The drawing under review shows one solid part. Ordinate dimensions are in mm from its lowest x, y, z. A direction names the side the tool comes from. Round coordinates to 2 decimals unless told otherwise and drop trailing zeros. Order: outer loops, then holes, each group sorted by start corner. A loop starts at its lowest first (then second) coordinate and runs counter-clockwise, first axis right, second up.
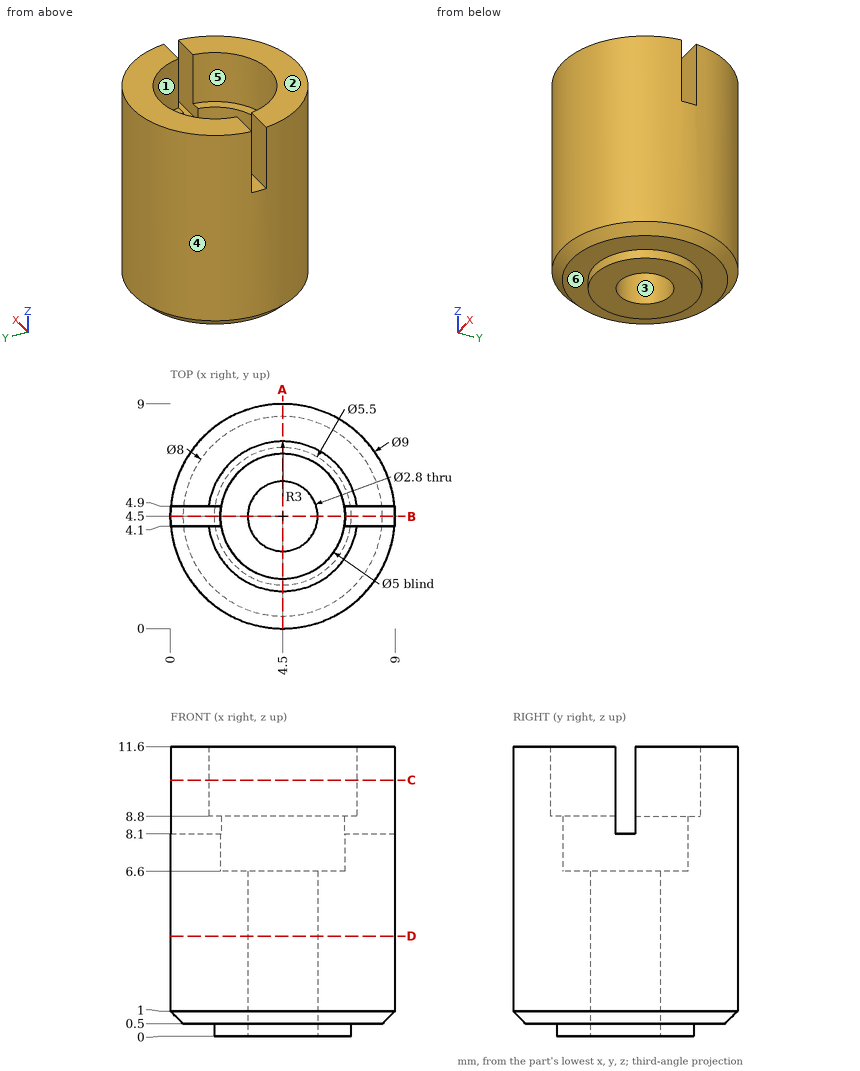
Q1. Wall thickness on line 1 (Y direction, x = 4.5, z = 7.5); line 2 (Y direction, x = 4.5, z = 3): over which ranges is each line inside the solid? List them lowest first.
Q2. Mouldability with a two-part tool opening along X and no side actions: class the marked faces 3, 4, 5 and 6 as +X half, -X half, draft (parallel to the pull), parting line (faces both ways), or undercut.
Q3. Take a section at B-B, the plane y = 4.5. State the section outline as (x, z) points.
Q4. Take a section at A-A, the plane x = 4.5. State the section outline as (y, z) points, plus the area to 3 significant figures.
Q5. Clearance check with flat-ended pins moving along their axes: pin 1 (1 mm diameter, centred on x = 8, z = 9, fed in from -Y); pin 2 (4 mm diameter, centred on y = 2.5, z = 9.5, fed in from +X); pin 3 (1.3 mm diameter, centred on x = 4.5, y = 3.5, fed in from +Z); pin 4 (1.5 mm diameter, centred on x = 4.5, y = 4, fed in from +Z). State where each tip first meets the part, or that it passes through.
Q6. Tool access review of the marked faces 1 and 2: name each direction out of +Z, -Z, +X, -X, +Y, -Y from which nothing blocks a thin tool from reaching the whole face with its end or side.
Q7. Take a section at D-D, the plane z = 4. State the section outline as (x, y) points.
Q8. Take a section at C-C, the plane z = 10.25. State the section outline as (x, y) points.
Working result:
1. line 1: y = 0 to 2, 7 to 9
1. line 2: y = 0 to 3.1, 5.9 to 9
2. face 3: undercut
2. face 4: parting line
2. face 5: undercut
2. face 6: draft
3. outline: (0, 1) - (0.5, 0.5) - (1.75, 0.5) - (1.75, 0) - (3.1, 0) - (3.1, 6.6) - (2, 6.6) - (2, 8.1) - (0, 8.1) - close; (5.9, 0) - (7.25, 0) - (7.25, 0.5) - (8.5, 0.5) - (9, 1) - (9, 8.1) - (7, 8.1) - (7, 6.6) - (5.9, 6.6) - close
4. outline: (0, 1) - (0.5, 0.5) - (1.75, 0.5) - (1.75, 0) - (3.1, 0) - (3.1, 6.6) - (2, 6.6) - (2, 8.8) - (1.5, 8.8) - (1.5, 11.6) - (0, 11.6) - close; (5.9, 0) - (7.25, 0) - (7.25, 0.5) - (8.5, 0.5) - (9, 1) - (9, 11.6) - (7.5, 11.6) - (7.5, 8.8) - (7, 8.8) - (7, 6.6) - (5.9, 6.6) - close
4. area: 56.1 mm2
5. pin 1: stops at y = 1.15
5. pin 2: stops at x = 8.98
5. pin 3: stops at z = 6.6
5. pin 4: passes through
6. face 1: +Z
6. face 2: +Z, +X, -X, +Y, -Y
7. outline: circle Ø9 at (4.5, 4.5); hole circle Ø2.8 at (4.5, 4.5)
8. outline: (0.02, 4.1) arc R4.5 ccw to (8.98, 4.1) - (7.47, 4.1) arc R3 cw to (1.53, 4.1) - close; (0.02, 4.9) - (1.53, 4.9) arc R3 cw to (7.47, 4.9) - (8.98, 4.9) arc R4.5 ccw to start
